Check sheet for the drawn part. Datum: minimum x, y, z corner. Units: mm. A direction names the side the tool comes from. Give positions to 0.01 mm unless a question says otherwise; leave off trailing zeros. Order: outer loops, then holes, each group sorted by start corner. A loop starts at its lowest first (then second) coordinate and runs counter-clockwise, first axis right, second up. Notation, with made-up numbers: (47, 88) -> (58, 88) arc R27 ccw to (58, 119) -> close; hole circle Ø3 at (-26.75, -11.5). An arc over 180 degrees is marked (long way). Return JSON: item names as keys, results as strings. Group by question number.
(1) Release check for a two-part mould opening along X. For the marked faces 1, 2 and 3 record: pulls with the +X half, pulls with the -X half, needs draft (parallel to the pull), parting line crosses it, or undercut.
(2) Cross-section at B-B on z = 6. Enter the section's corners in (x, y), then the cut area to 3 significant figures.
(3) Cross-section at D-D on y = 1. Enter the section's corners in (x, z).
(4) Cross-section at A-A on x = 6. Enter the section's corners in (y, z), then the cut area to 3 significant figures.
(5) Tool access check on the marked faces 4 and 5. Record the directions out of +Z, -Z, +X, -X, +Y, -Y that give a thin tool (end or side, any length) a straight path to the whole face; none if there is none.
(6) Thickness scan on line 1 along X through (y, z) = (10.25, 6); line 2 along X through (y, z) = (6.5, 6); line 3 along Z through (x, y) = (8.5, 9.5). Record the ranges inside material, lowest first.
(7) Depth check by flat-ended pin: pin 1 Ø1 at (x, y) = (4.5, 5.5) entering from -Z; pin 2 Ø2.5 at (x, z) = (6, 6) entering from -Y; pin 3 Ø3 at (y, z) = (4.5, 9) entering from -X; pin 4 Ø5 at (y, z) = (5.5, 1.5) entering from -X. Enter the tip coordinate at first touch or a pass-through.
(8) Cross-section at C-C on y = 6.5. Enter the section's corners in (x, z).
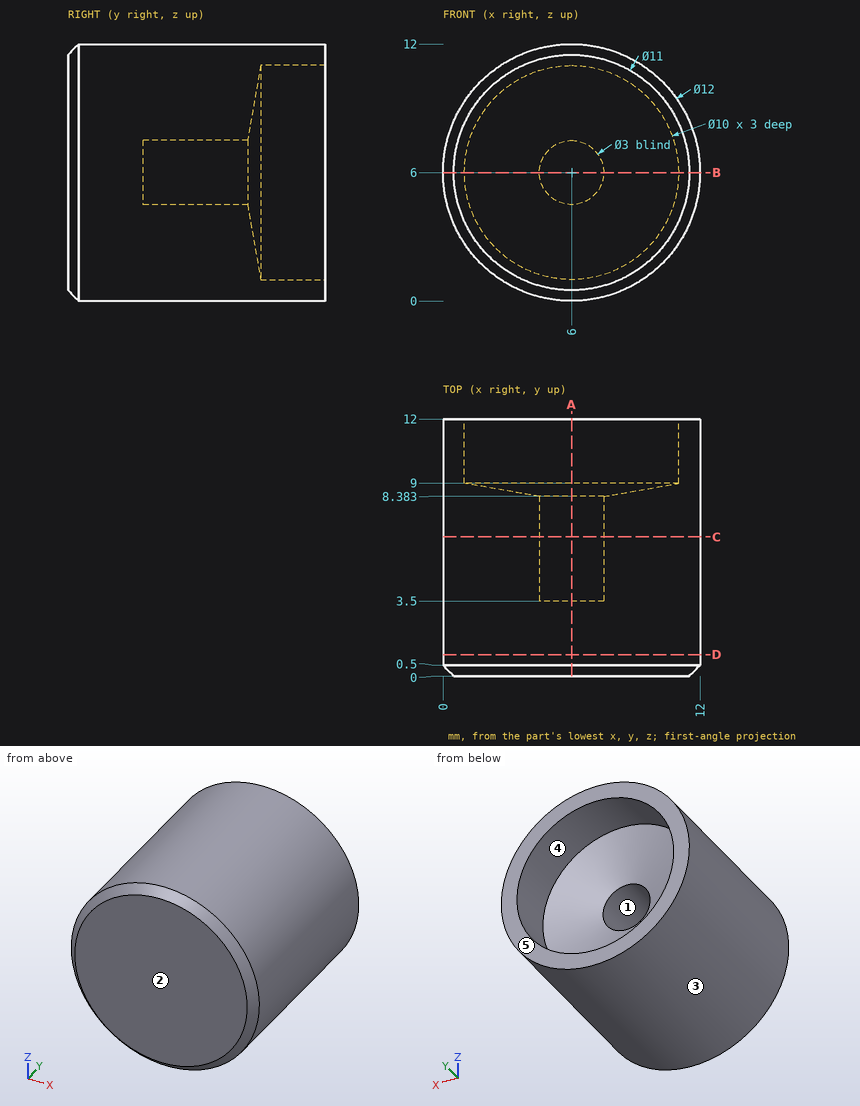
Verdict:
{
 "1": {"face 1": "undercut", "face 2": "needs draft", "face 3": "parting line crosses it"},
 "2": {"outline": "(0, 0.5) -> (0.5, 0) -> (11.5, 0) -> (12, 0.5) -> (12, 12) -> (11, 12) -> (11, 9) -> (7.5, 8.38) -> (7.5, 3.5) -> (4.5, 3.5) -> (4.5, 8.38) -> (1, 9) -> (1, 12) -> (0, 12) -> close", "area": "95.1 mm²"},
 "3": {"outline": "circle Ø12 at (6, 6)"},
 "4": {"outline": "(0, 0.5) -> (0.5, 0) -> (12, 0) -> (12, 1) -> (9, 1) -> (8.38, 4.5) -> (3.5, 4.5) -> (3.5, 7.5) -> (8.38, 7.5) -> (9, 11) -> (12, 11) -> (12, 12) -> (0.5, 12) -> (0, 11.5) -> close", "area": "95.1 mm²"},
 "5": {"face 4": "+Y", "face 5": "+Z, -Z, +X, -X, +Y"},
 "6": {"line 1": "0 to 1, 11 to 12", "line 2": "0 to 4.5, 7.5 to 12", "line 3": "0.55 to 1.67, 10.33 to 11.45"},
 "7": {"pin 1": "z = 0.08", "pin 2": "y = 0", "pin 3": "x = 0.19", "pin 4": "x = 0.34"},
 "8": {"outline": "circle Ø12 at (6, 6); hole circle Ø3 at (6, 6)"}
}
